Could you check a few things on this model? Use its own coordinates, in mm. A direction names the side the tool comes from. Round coordinates to 2 decimals unless told otherwise and drop trailing zeros. Write each loop counter-clockwise with the first axis right and the second up, starting at its lowest first coordinate (ties: lowest second). Pieces come first, ordered by that corner, then holes. Notation, with made-up numbers: (27, 84) -> (75, 84) arc R22 cw to (75, 122) -> close; hole circle Ø3 at (18, 55). An arc over 180 degrees is marked (long way). Return JSON: item names as keys, results as strings.
Autodesk Inventor part; units mm, degrees
ref_plane "作業平面1" through (0, 0, -400) normal (0, 0, 1) x (1, 0, 0)
sketch "スケッチ3" plane through (0, 0, 0) normal (0, 0, 1) x (1, 0, 0)
  circle A0 centre (0, 0) radius 25
  dimension "d7" = 50
extrude "押し出し2" add sketch "スケッチ3" against normal blind 400
sketch "スケッチ4" plane through (0, 0, 0) normal (0, 1, 0) x (-1, 0, 0)
  circle A0 centre (0, 0) radius 25
  dimension "d10" = 50
extrude "押し出し3" add sketch "スケッチ4" along normal mid plane 75
sketch "スケッチ5" plane through (0, -37.5, 0) normal (0, -1, 0) x (1, 0, 0)
  circle A0 centre (0, 0) radius 20
  dimension "d13" = 40
extrude "押し出し4" cut sketch "スケッチ5" against normal blind 75
sketch "スケッチ6" plane through (0, 0, 0) normal (1, 0, 0) x (0, 1, 0)
  circle A0 centre (0, -400) radius 15
  line L0 (-52.5, 0) -> (52.5, 0)
  point P0 (0, 0)
  dimension "d16" = 30
  dimension "d17" = 400
extrude "押し出し5" add sketch "スケッチ6" along normal mid plane 75
properties part number "LowerlegP"
1) For faces 4 (the face through (5.42, -0.525, 24.406)), 5 (the face through (0, -19, -400)), 6 (the face through (11, 37.5, 17)), which set-ups out of +Z, -Z, +X, -X, +Y, -Y let a thin tool reach every point of the face, with its end or its side?
Return value:
{"face 4": "none", "face 5": "-Z, +X, -X, -Y", "face 6": "+Z, -Z, +X, -X, +Y"}
2) Thinking about a two-plate mould opening in Z: for faces 1 (the face through (-37.5, 0, -400)), 2 (the face through (-24.976, 1.099, -197.2)), 3 (the face through (0, 19, -400)), which applies, pulls with the +Z half, pulls with the -Z half, needs draft (parallel to the pull), parting line crosses it, or undercut?
Return value:
{"face 1": "needs draft", "face 2": "undercut", "face 3": "pulls with the -Z half"}
3) I want a section at D-D, the plane z = -212. Please give me the cut outline in (x, y).
Return value:
{"outline": "circle Ø50 at (0, 0)"}
4) I want a section at A-A, the plane x = 0. Please give me the cut outline in (y, z).
Return value:
{"outline": "(-37.5, -25) -> (-25, -25) -> (-25, -400) -> (-15, -400) arc R15 ccw to (15, -400) -> (25, -400) -> (25, -25) -> (37.5, -25) -> (37.5, -20) -> (-37.5, -20) -> close; (-37.5, 20) -> (37.5, 20) -> (37.5, 25) -> (-37.5, 25) -> close"}
5) I want a section at B-B, the plane y = 0. Please give me the cut outline in (x, z), and give its area (3 significant figures).
Return value:
{"outline": "(-37.5, -415) -> (37.5, -415) -> (37.5, -385) -> (25, -385) -> (25, 0) arc R25 ccw to (-25, 0) -> (-25, -385) -> (-37.5, -385) -> close; hole circle Ø40 at (0, 0)", "area": "21,200 mm²"}
6) I want a section at C-C, the plane x = -30. Please give me the cut outline in (y, z).
Return value:
{"outline": "circle Ø30 at (0, -400)"}
7) If I drill on probe 1 along Z at (x, y) = (0, 1); probe 2 along Z at (x, y) = (0, 19); probe 3 along Y at (x, z) = (-20, -214.5), over which ranges is the centre line in solid material (lowest first)? Write a range as [from, to].
Return value:
{"probe 1": "[-414.97, -20], [20, 25]", "probe 2": "[-400, -20], [20, 25]", "probe 3": "[-15, 15]"}
8) Will these pins go through, and if not, where does the flat tip stop? pin 1 Ø8 at (x, y) = (2, -6) entering from +Z; pin 2 Ø3 at (x, y) = (-6, -22.5) entering from -Z; pin 3 Ø6 at (y, z) = (25.5, -92.5) entering from +X.
Return value:
{"pin 1": "z = 25", "pin 2": "z = -400", "pin 3": "x = 10.9"}
